Geometry check sheet. Reference: the model listing, model coordinates, mm. Round coordinates to 2 decimals unless told otherwise and drop trailing zeros.
(1) Cross-section at A-A on z = 7. Count the separate pieces of the cut face and the enclosed holes in it, and give its area (3 significant figures).
(2) Thickness scan on L1, parallel to Y at x = -376.5, z = 2; L2, parallel to X at y = -17, z = 8.5; L3, parallel to Y at x = -121.5, z = 5.25. Record the ranges inside material, lowest first.
(3) Gauge pin test, flat ends, axial feed: P1, Ø5, axis at y = -14.5, z = 2.5, coming from the -X side; P2, Ø3, axis at x = -692, z = 4.5, coming from the -Y side; P3, Ø3, axis at x = -204, z = 4, coming from the -Y side. Record the tip position at first contact, or that the pin passes through.
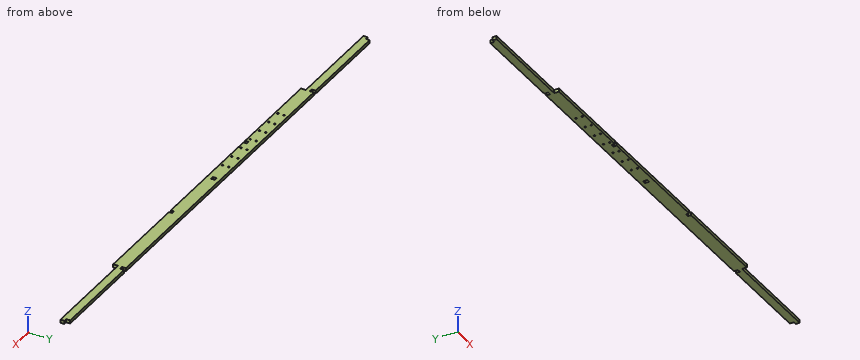
from build123d import *

# Parameters (mm, degrees)
SKETCH1_W           = 10.05
SKETCH1_H           = 12.5
BOSS_EXTRUDE1_DEPTH = 10
SKETCH2_R           = 2.5
CUT_EXTRUDE1_DEPTH  = 836.29934754


with BuildPart() as part:
    # Sketch1 → Boss-Extrude1 (new body)
    with BuildSketch(Plane.XY):
        Polygon((517.5, 20), (-517.5, 20), (-517.5, 7.5), (-527.5, 7.5), (-527.5, 20), (-825, 20), (-825, 7.5), (-835, 7.5), (-835, -5), (-517.5, -5), (-517.5, -20), (-210, -20), (-210, -10), (-200, -10), (-200, -20), (200, -20), (200, -10), (210, -10), (210, -20), (517.5, -20), (517.5, -5), (835, -5), (835, 7.5), (825, 7.5), (825, 20), (527.5, 20), (527.5, 7.5), (517.5, 7.5), align=None)
        with Locations((0.025, 1.25)):
            Rectangle(SKETCH1_W, SKETCH1_H, mode=Mode.SUBTRACT)
    extrude(amount=BOSS_EXTRUDE1_DEPTH)

    # Sketch2 → Cut-Extrude1 (cut, through all)
    with BuildSketch(Plane.XY.offset(10)):
        with Locations((-375.5, 7.3)):
            Circle(SKETCH2_R)
        with Locations((-375.5, -11.75)):
            Circle(SKETCH2_R)
        with Locations((-324.7, -11.75)):
            Circle(SKETCH2_R)
        with Locations((-324.7, 7.3)):
            Circle(SKETCH2_R)
        with Locations((-273.9, 7.3)):
            Circle(SKETCH2_R)
        with Locations((-273.9, -11.75)):
            Circle(SKETCH2_R)
        with Locations((-223.1, -11.75)):
            Circle(SKETCH2_R)
        with Locations((-223.1, 7.3)):
            Circle(SKETCH2_R)
        with Locations((-172.3, 7.3)):
            Circle(SKETCH2_R)
        with Locations((-121.5, -11.75)):
            Circle(SKETCH2_R)
        with Locations((-121.5, 7.3)):
            Circle(SKETCH2_R)
        with Locations((-70.7, 7.3)):
            Circle(SKETCH2_R)
        with Locations((-70.7, -11.75)):
            Circle(SKETCH2_R)
        with Locations((-172.3, -11.75)):
            Circle(SKETCH2_R)
    extrude(amount=-CUT_EXTRUDE1_DEPTH, mode=Mode.SUBTRACT)


solid = part.part
Found:
1. separate pieces: 1
1. enclosed holes: 15
1. area: 56,200 mm2
2. L1: y = -20 to -14.04, -9.46 to 5.01, 9.59 to 20
2. L2: x = -517.5 to -210, -200 to 200, 210 to 517.5
2. L3: y = -20 to -14.25, -9.25 to 4.8, 9.8 to 20
3. P1: stops at x = -517.5
3. P2: stops at y = -5
3. P3: stops at y = -10
